Model file for the job. Use its own axes, mm. A direction names the side the tool comes from. Give positions to 0.01 mm unless a question says otherwise; leave off trailing zeros. Loops run counter-clockwise (first coordinate to the right, second up) from the corner with the lowest first, then second, coordinate; pieces in that order, holes last. Notation, with made-up numbers: (84, 84) - (142, 84) arc R25 ccw to (142, 105) - close; hole circle Ø5 at (36, 58). An arc over 180 degrees is marked (long way). Answer as CSV lines item,"result". Start each with the question number.
Item 1: Tool access for faces 1 (the flat face through (-4, -23.59, -2)), 2 (the flat face through (-5.79, -15, -2)), 3 (the flat face through (27, 4, 1)): list every direction of +Z, -Z, +X, -X, +Y, -Y with a clear straight run to the whole face (end or side of a thin tool).
Item 2: Saw through at C-C on y = -19. Give the cut face in (x, z), plus the area to 3 significant figures.
Item 3: Pull direction Y, two halves, no side cores. Call faces 4 (the flat face through (0, -25, 1)), 5 (the flat face through (6, -27, 1)), 6 (the flat face through (-25, 0, 1)): pulls with the +Y half, pulls with the -Y half, needs draft (parallel to the pull), parting line crosses it, or undercut.
Item 4: Saw through at A-A on z = -3.75. Give the cut face in (x, y), plus the area to 3 significant figures.
Item 5: Saw through at D-D on x = -19. Give the cut face in (y, z), plus the area to 3 significant figures.
Item 6: Drill centre lines: L1, parallel to X at y = -19, z = 0.8; L2, parallel to Z at x = -12.5, y = 25. Where is each one in solid material? Low to high. Write a range as from..to.
Item 7: Pin check, flat tips, straight feed: pin 1 (1.3 mm diameter, centred on y = -14, z = -2.5, fed in from -X); pin 2 (0.5 mm diameter, centred on x = 26.5, z = 0.5, fed in from -Y); pin 3 (1 mm diameter, centred on x = -14, y = 14.5, fed in from +Z). Stop position of each tip, or through.
Item 8: Saw through at B-B on x = 3. Give the cut face in (y, z), plus the area to 3 significant figures.
from build123d import *

# Parameters (mm, degrees)
BOSS_EXTRUDE1_DEPTH = 1.6
SKETCH2_R           = 1.1
CUT_EXTRUDE1_DEPTH  = 42.839694072
SKETCH3_W           = 25.6
SKETCH3_H           = 2
BOSS_EXTRUDE2_DEPTH = 4.5
SKETCH4_W           = 20.8
SKETCH4_H           = 0.5
CUT_EXTRUDE2_DEPTH  = 2
SKETCH5_W           = 3.7
SKETCH5_H           = 17.2
SKETCH5_H_2         = 16.7
BOSS_EXTRUDE3_DEPTH = 4.5


with BuildPart() as part:
    # Sketch1 → Boss-Extrude1 (new body)
    with BuildSketch(Plane.XY):
        with BuildLine():
            Line((-6, 29.393876913), (-6, 25))
            Line((-6, 25), (6, 25))
            Line((6, 25), (6, 29.393876913))
            ThreePointArc((6, 29.393876913), (21.918226631, 20.483928855), (29.732137495, 4))
            Line((29.732137495, 4), (25, 4))
            Line((25, 4), (25, -4))
            Line((25, -4), (29.732137495, -4))
            ThreePointArc((29.732137495, -4), (21.918226631, -20.483928855), (6, -29.393876913))
            Line((6, -29.393876913), (6, -25))
            Line((6, -25), (-6, -25))
            Line((-6, -25), (-6, -29.393876913))
            ThreePointArc((-6, -29.393876913), (-21.918226631, -20.483928855), (-29.732137495, -4))
            Line((-29.732137495, -4), (-25, -4))
            Line((-25, -4), (-25, 4))
            Line((-25, 4), (-29.732137495, 4))
            ThreePointArc((-29.732137495, 4), (-21.918226631, 20.483928855), (-6, 29.393876913))
        make_face()
    extrude(amount=BOSS_EXTRUDE1_DEPTH)

    # Sketch2 → Cut-Extrude1 (cut, through all)
    with BuildSketch(Plane.XY):
        with Locations((-19, 19)):
            Circle(SKETCH2_R)
        with Locations((19, 19)):
            Circle(SKETCH2_R)
        with Locations((19, -19)):
            Circle(SKETCH2_R)
        with Locations((-19, -19)):
            Circle(SKETCH2_R)
    extrude(amount=CUT_EXTRUDE1_DEPTH, mode=Mode.SUBTRACT)

    # Sketch3 → Boss-Extrude2 (add)
    with BuildSketch(Plane.XY.offset(1.6)):
        with Locations((-2.5, 22.2)):
            Rectangle(SKETCH3_W, SKETCH3_H)
    extrude(amount=BOSS_EXTRUDE2_DEPTH)

    # Sketch4 → Cut-Extrude2 (cut)
    with BuildSketch(Plane.XY.offset(6.1)):
        with Locations((-2.5, 21.95)):
            Rectangle(SKETCH4_W, SKETCH4_H)
    extrude(amount=-CUT_EXTRUDE2_DEPTH, mode=Mode.SUBTRACT)

    # Sketch5 → Boss-Extrude3 (add)
    with BuildSketch(Plane(origin=(0, 0, 0), x_dir=(-1, 0, 0), z_dir=(0, 0, -1))):
        with Locations((-6.75, -3.81)):
            Rectangle(SKETCH5_W, SKETCH5_H)
        with Locations((3.94, -15.24)):
            Rectangle(SKETCH5_W, SKETCH5_H_2)
    extrude(amount=BOSS_EXTRUDE3_DEPTH)


solid = part.part
Responses:
1,face 1,"-Z, +X, -X, -Y"
1,face 2,"-Z, -X, +Y, -Y"
1,face 3,"+Z, -Z, +X"
2,outline,"(-23.22, 0) - (-20.1, 0) - (-20.1, 1.6) - (-23.22, 1.6) - close; (-17.9, 0) - (-5.79, 0) - (-5.79, -4.5) - (-2.09, -4.5) - (-2.09, 0) - (17.9, 0) - (17.9, 1.6) - (-17.9, 1.6) - close; (20.1, 0) - (23.22, 0) - (23.22, 1.6) - (20.1, 1.6) - close"
2,area,"83.9 mm2"
3,face 4,"pulls with the -Y half"
3,face 5,"needs draft"
3,face 6,"undercut"
4,outline,"(-5.79, -23.59) - (-2.09, -23.59) - (-2.09, -6.89) - (-5.79, -6.89) - close; (4.9, -12.41) - (8.6, -12.41) - (8.6, 4.79) - (4.9, 4.79) - close"
4,area,"125 mm2"
5,outline,"(-23.22, 0) - (-20.1, 0) - (-20.1, 1.6) - (-23.22, 1.6) - close; (-17.9, 0) - (17.9, 0) - (17.9, 1.6) - (-17.9, 1.6) - close; (20.1, 0) - (23.22, 0) - (23.22, 1.6) - (20.1, 1.6) - close"
5,area,"67.3 mm2"
6,L1,"-23.22..-20.1, -17.9..17.9, 20.1..23.22"
6,L2,"0..1.6"
7,pin 1,"x = -5.79"
7,pin 2,"y = -14.52"
7,pin 3,"z = 1.6"
8,outline,"(-25, 0) - (25, 0) - (25, 1.6) - (23.2, 1.6) - (23.2, 6.1) - (22.2, 6.1) - (22.2, 4.1) - (21.7, 4.1) - (21.7, 6.1) - (21.2, 6.1) - (21.2, 1.6) - (-25, 1.6) - close"
8,area,"88.0 mm2"
